Geometry: final body of the model. Coordinates: model frame, mm. A direction names the side the tool comes from. Give positions to 0.01 mm unless a question says otherwise; leave off trailing zeros. Loops run counter-clockwise (first coordinate to the right, second up) from the corner with the lowest first, then second, coordinate; pieces in that order, holes last. Notation, with made-up numbers: (66, 15.5) -> (117, 15.5) arc R27 ccw to (117, 54.5) -> close; hole circle Ø10 at (20, 62.25). An arc over 180 degrees is marked (long way). Answer in a Markdown table with one row per item. Add a question column.
from build123d import *

# Parameters (mm, degrees)
F1_DEPTH = 10
F2_R     = 0.5
F3_DEPTH = 240
F5_DEPTH = 20


with BuildPart() as f1:
    # F0 (on Front) → F1 (new body)
    with BuildSketch(Plane.XZ):
        Polygon((82.249313, 125.919251), (142.249313, 125.919251), (142.249313, -114.080749), (82.249313, -114.080749), (82.249313, -144.080749), (142.249313, -144.080749), (242.249313, -144.080749), (242.249313, 155.919251), (142.249313, 155.919251), (82.249313, 155.919251), align=None)
    extrude(amount=F1_DEPTH)

    # F2 (on face) → F3 (join, through all)
    with BuildSketch(Plane.XY.offset(-114.080749)):
        with Locations((87.249313, -5)):
            Circle(F2_R)
    extrude(amount=F3_DEPTH)

    # F4 (on face) → F5 (join)
    with BuildSketch(Plane.XZ.offset(10)):
        with BuildLine():
            ThreePointArc((208.744351, 103.722573), (204.638161, 109.479239), (198.881495, 105.373049))
            Line((198.881495, 105.373049), (165.871974, -91.884072))
            ThreePointArc((165.871974, -91.884072), (169.978164, -97.640738), (175.73483, -93.534548))
            Line((175.73483, -93.534548), (208.744351, 103.722573))
        make_face()
    extrude(amount=-F5_DEPTH)


solid = f1.part
(1) Cut plane C-C on x = 216.5. Return the cut outline in (y, z).
(2) Draft query along Z for faces 4 (the flat face through (113, -5, -114.081)), 5 (the flat face through (242.249, -5, 4)), 6 (the flat face through (192.01, 4.93, 3.71)), 7 (the flat face through (112, -5, 125.919)). Return one class per face: +Z half, -Z half, draft (parallel to the pull), parting line (faces both ways), or undercut.
(3) Pin query (flat end, axial travel): pin 1 Ø5 at (y, z) = (7, 111.5) entering from +X; pin 2 Ø1.5 at (y, z) = (-0.5, 78) entering from -X. Return the tip coordinate at first contact, or that it passes through.
(4) Cut plane A-A on x = 101. Return the cut outline in (y, z), then the cut area to 3 significant figures.
(5) Material intervals for line 1 along Z through (x, y) = (122, -8.25); line 2 along Y through (x, z) = (172, 129); line 3 along X through (y, z) = (-7.5, 123), sorted ascending. Write a range as from..to.
(6) Cut plane B-B on z = 21. Return the cut outline in (x, y).
(7) Cut plane D-D on x = 179. Return the cut outline in (y, z).
(8) Reachability of faces 1 (the flat face through (163, -5, 155.919)), 2 (the flat face through (179, 0, 8)), 3 (the flat face through (182.61, 4.93, 8.13)) from +Z, -Z, +X, -X, +Y, -Y: full face, straight path, thin tool, end or side. Return the list, or none.
Answer list:
| question | item | result |
|---|---|---|
| 1 | outline | (-10, -144.08) -> (0, -144.08) -> (0, 155.92) -> (-10, 155.92) -> close |
| 2 | face 4 | undercut |
| 2 | face 5 | draft |
| 2 | face 6 | -Z half |
| 2 | face 7 | undercut |
| 3 | pin 1 | stops at x = 206.09 |
| 3 | pin 2 | stops at x = 142.25 |
| 4 | outline | (-10, -144.08) -> (0, -144.08) -> (0, -114.08) -> (-10, -114.08) -> close; (-10, 125.92) -> (0, 125.92) -> (0, 155.92) -> (-10, 155.92) -> close |
| 4 | area | 600 mm² |
| 5 | line 1 | z = -144.08..-114.08, 125.92..155.92 |
| 5 | line 2 | y = -10..0 |
| 5 | line 3 | x = 142.25..242.25 |
| 6 | outline | circle Ø1 at (87.25, -5); (142.25, -10) -> (242.25, -10) -> (242.25, 0) -> (194.9, 0) -> (194.9, 10) -> (184.76, 10) -> (184.76, 0) -> (142.25, 0) -> close |
| 7 | outline | (-10, -144.08) -> (0, -144.08) -> (0, -74.02) -> (10, -74.02) -> (10, -13.43) -> (0, -13.43) -> (0, 155.92) -> (-10, 155.92) -> close |
| 8 | face 1 | +Z, +X, -X, +Y, -Y |
| 8 | face 2 | +Y |
| 8 | face 3 | +Z, -X, +Y |
